CAD build for the part. Positions are in the model's coordinates, mm. A direction names the side the tool comes from. Give positions to 0.01 mm unless a question says otherwise; leave off trailing zeros. Write each loop counter-clockwise with the first axis right and the second up, starting at its lowest first coordinate (ties: lowest second). Pieces come first, ordered by that corner, then holes. Notation, with made-up numbers: (69, 1) - (88, 1) arc R27 ccw to (88, 37) - close; hole circle Ø10 at (54.25, 8.25). An arc over 180 degrees is marked (long way). Put each result on its own line as item: value. Start each with the question number.
1. Wall check: line 1 (Y direction, x = 0, z = 4.1); line 2 (Z direction, x = -17, y = 3) (3 decimals); line 3 (Y direction, x = -13.5, z = 0.8). Give the ranges that are in metal, low to high.
2. Cut at C-C on x = 12. List the corners of the cut face in (y, z) (3 decimals).
3. Mould opens along Y. For faces 6 (the flat face through (3, -1, 4.978)), 7 (the cylindrical face through (-2.182, -1.673, 3.42)), 8 (the flat face through (0, 19.253, 1)), 9 (the cylindrical face through (-0.115, -16.124, 0.939)) say: +Y half, -Y half, draft (parallel to the pull), parting line (faces both ways), or undercut.
4. Cut at A-A on y = 0. Give the number of separate pieces and of enclosed holes in the cut face, and give its area (3 significant figures).
5. Drop flat-ended pins along their axis: pin 1 (1.5 mm diameter, centred on x = -10, z = 1.5, fed in from +Y); pin 2 (2.5 mm diameter, centred on x = 0, y = 7.13, fed in from -Z); pin 3 (5 mm diameter, centred on x = -2, y = 7, fed in from +Z) (3 decimals); pin 4 (1.4 mm diameter, centred on x = 17, y = 0, fed in from +Z). Give the stop position or say it passes through.
6. Tool access for faces 1 (the flat face through (-12, 4.166, 1)), 2 (the flat face through (-4.4, 0.1, 1.905)), 3 (the flat face through (12, -4.166, 1)), 4 (the cylindrical face through (2.86, 0.9, -0.41)), 5 (the cylindrical face through (-0.115, 14.585, 0.939)): list every direction of +Z, -Z, +X, -X, +Y, -Y with a clear straight run to the whole face (end or side of a thin tool).
from build123d import *

# Parameters (mm, degrees)
F0_W     = 8.3312
F0_H     = 15.0876
F0_R     = 0.88265
F0_W_2   = 15.0876
F0_H_2   = 8.3312
F0_R_2   = 4.09575
F0_R_3   = 2.74955
F1_DEPTH = 1.905
F2_R     = 4.09575
F2_R_2   = 2.74955
F3_DEPTH = 3.0734
F4_R     = 3.5052
F4_R_2   = 2.9972
F5_DEPTH = 0.8255


with BuildPart() as f1:
    # F0 (on Top) → F1 (new body)
    with BuildSketch(Plane.XY):
        with Locations((0, 11.7094)):
            Rectangle(F0_W, F0_H)
        with Locations((0, 7.13105)):
            Circle(F0_R, mode=Mode.SUBTRACT)
        with Locations((0, 10.42035)):
            Circle(F0_R, mode=Mode.SUBTRACT)
        with Locations((0, 13.70965)):
            Circle(F0_R, mode=Mode.SUBTRACT)
        with Locations((0, 16.99895)):
            Circle(F0_R, mode=Mode.SUBTRACT)
        with Locations((11.7094, 0)):
            Rectangle(F0_W_2, F0_H_2)
        with Locations((7.13105, 0)):
            Circle(F0_R, mode=Mode.SUBTRACT)
        with Locations((10.42035, 0)):
            Circle(F0_R, mode=Mode.SUBTRACT)
        with Locations((13.70965, 0)):
            Circle(F0_R, mode=Mode.SUBTRACT)
        with Locations((16.99895, 0)):
            Circle(F0_R, mode=Mode.SUBTRACT)
        Rectangle(F0_W, F0_H_2)
        Circle(F0_R_2, mode=Mode.SUBTRACT)
        with Locations((-11.7094, 0)):
            Rectangle(F0_W_2, F0_H_2)
        with Locations((-16.99895, 0)):
            Circle(F0_R, mode=Mode.SUBTRACT)
        with Locations((-13.70965, 0)):
            Circle(F0_R, mode=Mode.SUBTRACT)
        with Locations((-10.42035, 0)):
            Circle(F0_R, mode=Mode.SUBTRACT)
        with Locations((-7.13105, 0)):
            Circle(F0_R, mode=Mode.SUBTRACT)
        with Locations((0, -11.7094)):
            Rectangle(F0_W, F0_H)
        with Locations((0, -16.99895)):
            Circle(F0_R, mode=Mode.SUBTRACT)
        with Locations((0, -13.70965)):
            Circle(F0_R, mode=Mode.SUBTRACT)
        with Locations((0, -10.42035)):
            Circle(F0_R, mode=Mode.SUBTRACT)
        with Locations((0, -7.13105)):
            Circle(F0_R, mode=Mode.SUBTRACT)
        Circle(F0_R_2)
        Circle(F0_R_3, mode=Mode.SUBTRACT)
        Circle(F0_R_3)
    extrude(amount=F1_DEPTH)

    # F2 (on face) → F3 (join)
    with BuildSketch(Plane.XY.offset(1.905)):
        Circle(F2_R)
        Circle(F2_R_2, mode=Mode.SUBTRACT)
    extrude(amount=F3_DEPTH)

    # F4 (on face) → F5 (join)
    with BuildSketch(Plane.XY):
        Circle(F4_R)
        Circle(F4_R_2, mode=Mode.SUBTRACT)
    extrude(amount=-F5_DEPTH)


solid = f1.part
Report:
1. line 1: y = -4.1 to -2.75, 2.75 to 4.1
1. line 2: z = 0 to 1.905
1. line 3: y = -4.17 to -0.86, 0.86 to 4.17
2. outline: (-4.166, 0) - (4.166, 0) - (4.166, 1.905) - (-4.166, 1.905) - close
3. face 6: draft
3. face 7: undercut
3. face 8: +Y half
3. face 9: undercut
4. separate pieces: 9
4. enclosed holes: 0
4. area: 55.6 mm²
5. pin 1: stops at y = 4.17
5. pin 2: stops at z = 0
5. pin 3: stops at z = 1.905
5. pin 4: passes through
6. face 1: +Z, -Z, -X, +Y
6. face 2: +Z
6. face 3: +Z, -Z, +X, -Y
6. face 4: -Z
6. face 5: +Z, -Z
